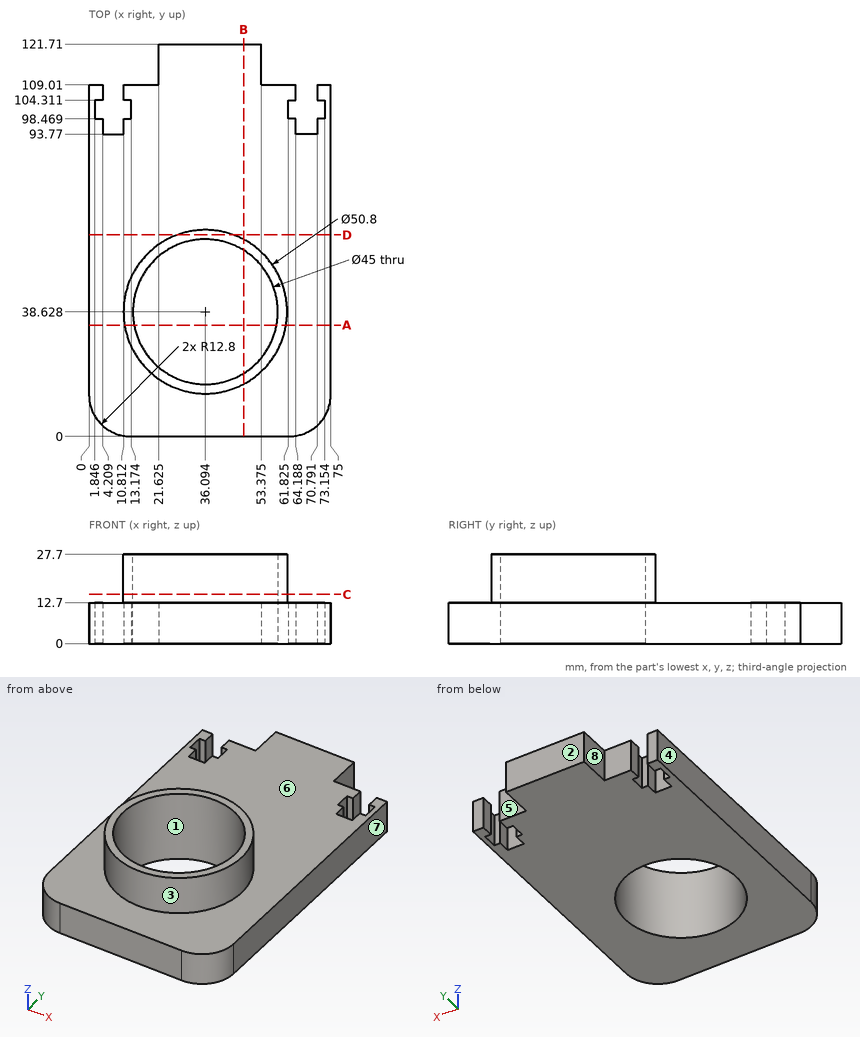
Design review of the part shown in the three views and the two pictorial views. Dimensions are in mm from the part's minimum x, y and z. A direction names the side the tool comes from. Coordinates: 2 decimals unless noted, no trailing zeros. Order: outer loops, then holes, each group sorted by start corner. A loop starts at its lowest first (then second) coordinate and runs counter-clockwise, first axis right, second up. Notation, with made-up numbers: (24, 18) - (48, 18) arc R22 cw to (48, 29) - close; hole circle Ø3 at (46, -37). An arc over 180 degrees is marked (long way). Answer as CSV lines item,"result". Start each with the question number.
1) Insertion check: P1, Ø2, axis at y = 80, z = 14, coming from the -X side; P2, Ø1.2, axis at x = 63, z = 4, coming from the -Y side; P3, Ø1, axis at y = 59, z = 18, coming from the +X side (1 decimal); P4, Ø1.9, axis at x = 3, z = 7, coming from the +Y side. Each pin has a flat end and moves straight along its axis. Give the tip position at first contact, or say it passes through.
2) Add section A-A (y = 34.5). State the section outline as (x, z) points (1 decimal), then the cut area to 3 significant figures.
3) Add section B-B (x = 48). State the section outline as (y, z) points (1 decimal), then the cut area to 3 significant figures.
4) Add section C-C (z = 15.25). State the section outline as (x, y) points.
5) To check wall thickness, follow line 1 along Z through (x, y) = (50.5, 101); line 2 along X through (y, z) = (116, 10) (1 decimal); line 3 along X through (y, z) = (57.5, 3.25) (1 decimal). State the ranges of each line that lie inside material, in increasing order. Write a range as [from, to].
6) Draft analysis for pull direction X (two halves, no side actions). For the marked faces 1, 2, 3 and 4, state which applies: +X half, -X half, draft (parallel to the pull), parting line (faces both ways), or undercut.
7) Add section D-D (y = 62.5). State the section outline as (x, z) points, then the cut area to 3 significant figures.
8) Machinability: for the marked faces 5, 6, 7 and 8, which of the approach directions +Z, -Z, +X, -X, +Y, -Y give a long, thin tool a straight path to every point of the face, cutting with its end or side? Answer none if there is none.
Result:
1,P1,"through"
1,P2,"y = 0"
1,P3,"x = 51.9"
1,P4,"y = 109.01"
2,outline,"(0, 0) - (14, 0) - (14, 27.7) - (11, 27.7) - (11, 12.7) - (0, 12.7) - close; (58.2, 0) - (75, 0) - (75, 12.7) - (61.2, 12.7) - (61.2, 27.7) - (58.2, 27.7) - close"
2,area,"479 mm^2"
3,outline,"(0, 0) - (19.5, 0) - (19.5, 27.7) - (16.2, 27.7) - (16.2, 12.7) - (0, 12.7) - close; (57.7, 0) - (121.7, 0) - (121.7, 12.7) - (61.1, 12.7) - (61.1, 27.7) - (57.7, 27.7) - close"
3,area,"1,160 mm^2"
4,outline,"circle Ø50.8 at (36.09, 38.63); hole circle Ø45 at (36.09, 38.63)"
5,line 1,"[0, 12.7]"
5,line 2,"[21.6, 53.4]"
5,line 3,"[0, 23.8], [48.3, 75]"
6,face 1,"undercut"
6,face 2,"draft"
6,face 3,"parting line"
6,face 4,"-X half"
7,outline,"(0, 0) - (75, 0) - (75, 12.7) - (44.77, 12.7) - (44.77, 27.7) - (27.42, 27.7) - (27.42, 12.7) - (0, 12.7) - close"
7,area,"1,210 mm^2"
8,face 5,"+Z, -Z, +X, +Y"
8,face 6,"+Z"
8,face 7,"+Z, -Z, +X, +Y, -Y"
8,face 8,"+Z, -Z, -X, +Y"
